Verification items for this drawing (mm, ordinates from the low corner). Give positions to 0.01 mm unless a question says otherwise; leave off trailing zeros. Loops run counter-clockwise (first coordinate to the right, second up) from the corner with the lowest first, then second, coordinate; pieces in that order, holes last. Notation, with made-up numbers: M -8.75,7 L 13.25,7 A26 ccw 13.25,38 Z; hole C 10.5,32.5 d8. An arc over 180 degrees is marked long. Answer in a Markdown table with one row per item.
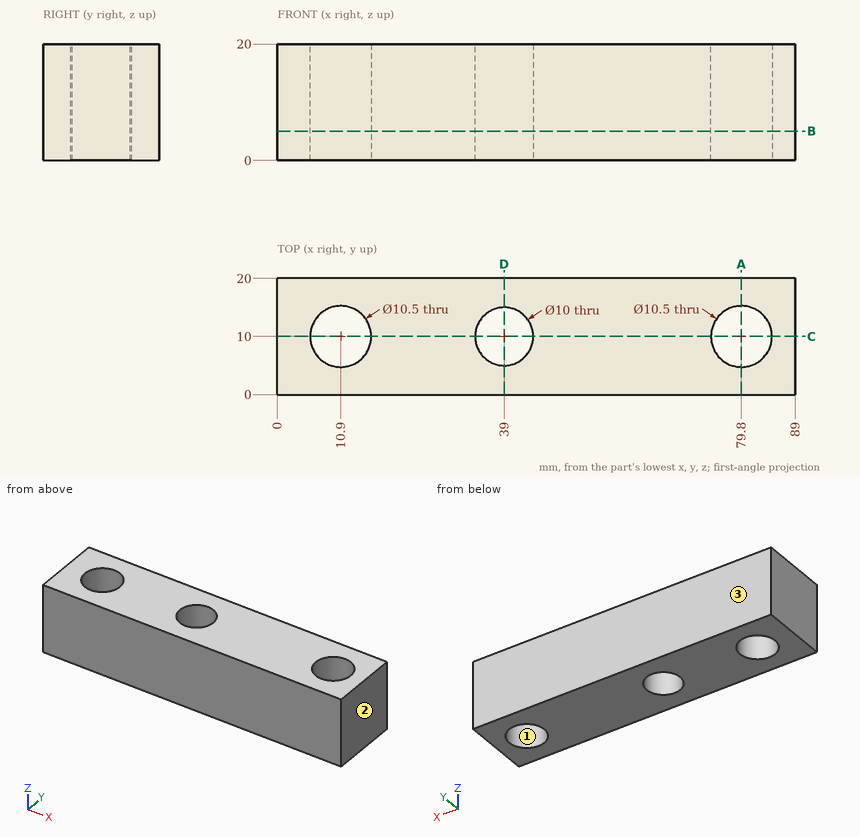
Item 1: Release check for a two-part mould opening along X. For the marked faces 1, 2 and 3 record: released by +X, released by -X, zero draft, split by the parting line, or undercut.
Reported:
| item | result |
|---|---|
| face 1 | undercut |
| face 2 | released by +X |
| face 3 | zero draft |
Item 2: Sectioned sample at C-C (y = 10). Record the cut outline in (x, z), and give its area (3 significant figures).
Reported:
| item | result |
|---|---|
| outline | M 0,0 L 5.65,0 L 5.65,20 L 0,20 Z; M 16.15,0 L 34,0 L 34,20 L 16.15,20 Z; M 44,0 L 74.55,0 L 74.55,20 L 44,20 Z; M 85.05,0 L 89,0 L 89,20 L 85.05,20 Z |
| area | 1,160 mm^2 |
Item 3: Scan lines: L1, parallel to Y at x = 39, z = 6; L2, parallel to X at y = 9, z = 14.75; L3, parallel to X at y = 7.5, z = 19. Record each from-to range of solid material in increasing order. Write a range as [from, to].
Reported:
| item | result |
|---|---|
| L1 | y = [0, 5], [15, 20] |
| L2 | x = [0, 5.75], [16.05, 34.1], [43.9, 74.65], [84.95, 89] |
| L3 | x = [0, 6.28], [15.52, 34.67], [43.33, 75.18], [84.42, 89] |
Item 4: Sectioned sample at B-B (z = 5). Record the cut outline in (x, y).
Reported:
| item | result |
|---|---|
| outline | M 0,0 L 89,0 L 89,20 L 0,20 Z; hole C 10.9,10 d10.5; hole C 39,10 d10; hole C 79.8,10 d10.5 |
Item 5: Sectioned sample at A-A (x = 79.8). Record the cut outline in (y, z), and give its area (3 significant figures).
Reported:
| item | result |
|---|---|
| outline | M 0,0 L 4.75,0 L 4.75,20 L 0,20 Z; M 15.25,0 L 20,0 L 20,20 L 15.25,20 Z |
| area | 190 mm^2 |
Item 6: Sectioned sample at D-D (x = 39). Record the cut outline in (y, z).
Reported:
| item | result |
|---|---|
| outline | M 0,0 L 5,0 L 5,20 L 0,20 Z; M 15,0 L 20,0 L 20,20 L 15,20 Z |
